Check sheet for the modelled part. Datum: model origin and axes. Units: mm. A direction names the side the tool comes from. Give positions to 0.01 mm unless a question says otherwise; leave off trailing zeros. Loops run counter-clockwise (first coordinate to the right, second up) from the corner with the lowest first, then second, coordinate; pieces in that order, holes last. Notation, with made-up numbers: (-12.75, 38.25) -> (9.25, 38.25) arc R26 cw to (9.25, 56.25) -> close; hole circle Ø1 at (61, 26.25). An arc over 180 degrees is marked (long way). Answer as CSV lines item,"result". Start each with the question number.
(1) Release check for a two-part mould opening along Y. For faces 1 (the face through (-2, 0, -4)), 2 (the face through (30, 32, -230)), 3 (the face through (0, 70, -107)), 4 (the face through (-3.25, 26.57, -230.28)) record: pulls with the +Y half, pulls with the -Y half, needs draft (parallel to the pull), parting line crosses it, or undercut.
(2) Access from +Z, -Z, +X, -X, +Y, -Y to the whole of each face (thin tool, end or side, straight path). Record for faces 5 (the face through (-7, 27, -127.5)), 6 (the face through (-7, 27, 250)), 7 (the face through (-30, 33, 107)).
(3) Section check C-C on z = -6.5. Enter the section's corners in (x, y), plus the area to 3 significant figures.
(4) Section check B-B on z = 217. Enter the section's corners in (x, y).
(5) Material ranges on line 1 (Z direction, x = -1.5, y = 13); line 2 (Y direction, x = 0, z = -225); line 3 (Y direction, x = 2, z = -163.5), recorded low to high. Write a range as from..to.
(6) Section check A-A on x = 0. State how many separate pieces and enclosed holes the cut face has, plus the area to 3 significant figures.
(7) Gauge pin test, flat ends, axial feed: pin 1 Ø5 at (y, z) = (48.5, -215) entering from -X; pin 2 Ø12 at (x, z) = (-5.5, 183.5) entering from +Y; pin 3 Ø20 at (y, z) = (22.5, -234.5) entering from +X. Record the tip position at first contact, or that the pin passes through.
from build123d import *

# Parameters (mm, degrees)
SKETCH1_W               = 240
SKETCH1_H               = 600
EXTRUDE1_DEPTH          = 10
SKETCH2_R               = 15
EXTRUDE2_DEPTH          = 40
MIRROR2_COPY_1_SKETCH_R = 15
MIRROR2_COPY_1_DEPTH    = 40


with BuildPart() as part:
    # Sketch1 → Extrude1 (new body)
    with BuildSketch(Plane(origin=(0, 0, 0), x_dir=(1, 0, 0), z_dir=(0, 1, 0))):
        Rectangle(SKETCH1_W, SKETCH1_H)
    extrude(amount=EXTRUDE1_DEPTH)

    # Sketch2 → Extrude2 (add)
    with BuildSketch(Plane.XY.offset(250)):
        with BuildLine():
            Line((-30, 10), (30, 10))
            Line((30, 10), (30, 55))
            ThreePointArc((30, 55), (25.606601718, 65.606601718), (15, 70))
            Line((15, 70), (-15, 70))
            ThreePointArc((-15, 70), (-25.606601718, 65.606601718), (-30, 55))
            Line((-30, 55), (-30, 10))
        make_face()
        with Locations((0, 41.214252503)):
            Circle(SKETCH2_R, mode=Mode.SUBTRACT)
    extrude2 = extrude(amount=-EXTRUDE2_DEPTH)

    # Mirror1: Extrude2 across plane
    add(extrude2.mirror(Plane.XY.offset(168.75)))

    # Mirror2: Extrude2 across plane
    add(extrude2.mirror(Plane.XY))

    # Mirror2 copy 1 sketch → Mirror2 copy 1 (add)
    with BuildSketch(Plane.XY.offset(-87.5)):
        with BuildLine():
            Line((-30, 10), (30, 10))
            Line((30, 10), (30, 55))
            ThreePointArc((30, 55), (25.606601718, 65.606601718), (15, 70))
            Line((15, 70), (-15, 70))
            ThreePointArc((-15, 70), (-25.606601718, 65.606601718), (-30, 55))
            Line((-30, 55), (-30, 10))
        make_face()
        with Locations((0, 41.214252503)):
            Circle(MIRROR2_COPY_1_SKETCH_R, mode=Mode.SUBTRACT)
    extrude(amount=-MIRROR2_COPY_1_DEPTH)


solid = part.part
Working result:
1,face 1,"pulls with the -Y half"
1,face 2,"needs draft"
1,face 3,"pulls with the +Y half"
1,face 4,"undercut"
2,face 5,"+X, -X, +Y"
2,face 6,"+Z, +X, -X, +Y"
2,face 7,"+Z, -Z, -X, +Y"
3,outline,"(-120, 0) -> (120, 0) -> (120, 10) -> (-120, 10) -> close"
3,area,"2,400 mm^2"
4,outline,"(-120, 0) -> (120, 0) -> (120, 10) -> (30, 10) -> (30, 55) arc R15 ccw to (15, 70) -> (-15, 70) arc R15 ccw to (-30, 55) -> (-30, 10) -> (-120, 10) -> close; hole circle Ø30 at (0, 41.21)"
5,line 1,"z = -250..-210, -127.5..-87.5, 87.5..127.5, 210..250"
5,line 2,"y = 0..26.21, 56.21..70"
5,line 3,"y = 0..10"
6,separate pieces,"5"
6,enclosed holes,"0"
6,area,"10,800 mm^2"
7,pin 1,"stops at x = -30"
7,pin 2,"stops at y = 10"
7,pin 3,"stops at x = 30"
